Work out the finished part from the listing and answer in its coordinate system (mm). Face numbers are marked on the shaded views. A direction names the side the tool comes from. Coordinates: 2 decimals unless noted, no trailing zeros. Write each loop counter-clockwise with the first axis right and the second up, starting at its lowest first coordinate (ties: lowest second). Pieces come first, ordered by that corner, then holes. Notation, with made-up numbers: (40.25, 12) - (89.25, 12) arc R8 ccw to (89.25, 19) - close; hole circle Ø8 at (-34.5, -35). An arc over 180 degrees is marked (long way). One line per item, written item: value.
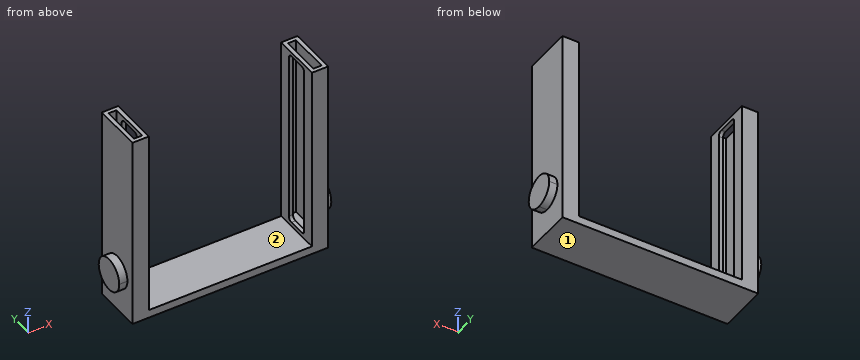
```python
from build123d import *

# Parameters (mm, degrees)
F0_W          = 25.4
F0_H          = 127
F1_DEPTH      = 31.75
F0_W_2        = 50.8
F0_H_2        = 152.4
F2_DEPTH      = 609.6
F0_W_3        = 508
F3_DEPTH      = 25.4
F4_DEPTH      = 609.6
F5_DEPTH      = 31.75
F6_W          = 76.2
F6_H          = 558.8
F7_DEPTH      = 25.4
F7_DEPTH_BACK = 533.4
F8_R          = 12.7
F10_DEPTH     = 25.4
F12_DEPTH     = 25.4


with BuildPart() as f1:
    # F0 (on Top) → F1 (new body)
    with BuildSketch(Plane.XY):
        with Locations((-80.5362447441, -59.7925535809)):
            Rectangle(F0_W, F0_H)
    extrude(amount=F1_DEPTH)

    # F0 (on Top) → F2 (join)
    with BuildSketch(Plane.XY):
        with Locations((-80.5362447441, -59.7925535809)):
            Rectangle(F0_W_2, F0_H_2)
        with Locations((-80.5362447441, -59.7925535809)):
            Rectangle(F0_W, F0_H, mode=Mode.SUBTRACT)
    extrude(amount=F2_DEPTH)

    # F0 (on Top) → F3 (join)
    with BuildSketch(Plane.XY):
        with Locations((198.8637552559, -59.7925535809)):
            Rectangle(F0_W_3, F0_H_2)
    extrude(amount=F3_DEPTH)

    # F0 (on Top) → F4 (join)
    with BuildSketch(Plane.XY):
        with Locations((478.2637552559, -59.7925535809)):
            Rectangle(F0_W_2, F0_H_2)
        with Locations((478.2637552559, -59.7925535809)):
            Rectangle(F0_W, F0_H, mode=Mode.SUBTRACT)
    extrude(amount=F4_DEPTH)

    # F0 (on Top) → F5 (join)
    with BuildSketch(Plane.XY):
        with Locations((478.2637552559, -59.7925535809)):
            Rectangle(F0_W, F0_H)
    extrude(amount=F5_DEPTH)

    # F6 (on face) → F7 (cut, two sides)
    with BuildSketch(Plane(origin=(452.8637552559, 0, 0), x_dir=(0, -1, 0), z_dir=(-1, 0, 0))) as f7_sk:
        with Locations((59.7925535809, 317.5)):
            Rectangle(F6_W, F6_H)
    extrude(amount=-F7_DEPTH, mode=Mode.SUBTRACT)
    extrude(f7_sk.sketch, amount=F7_DEPTH_BACK, mode=Mode.SUBTRACT)

    # F8
    f8_edges = [f1.edges().sort_by_distance(p)[0] for p in [
        (459.213755, -97.892554, 38.1),
        (459.213755, -21.692554, 38.1),
        (459.213755, -97.892554, 596.9),
        (459.213755, -21.692554, 596.9),
        (-61.486245, -21.692554, 38.1),
        (-61.486245, -21.692554, 596.9),
        (-61.486245, -97.892554, 596.9),
        (-61.486245, -97.892554, 38.1),
    ]]
    fillet(f8_edges, radius=F8_R)

    # F9 (on face) → F10 (join)
    with BuildSketch(Plane(origin=(-105.9362447441, 0, 0), x_dir=(0, -1, 0), z_dir=(-1, 0, 0))):
        with BuildLine():
            ThreePointArc((59.7925535809, 76.2), (95.7135780651, 91.0789755157), (110.5925535809, 127))
            ThreePointArc((110.5925535809, 127), (23.8715290966, 162.9210244843), (59.7925535809, 76.2))
        make_face()
    extrude(amount=F10_DEPTH)

    # F11 (on face) → F12 (join)
    with BuildSketch(Plane.YZ.offset(503.6637552559)):
        with BuildLine():
            ThreePointArc((-8.9925535809, 127), (-95.7135780651, 162.9210244843), (-59.7925535809, 76.2))
            ThreePointArc((-59.7925535809, 76.2), (-23.8715290966, 91.0789755157), (-8.9925535809, 127))
        make_face()
    extrude(amount=F12_DEPTH)


solid = f1.part
```
Item 1: Which of the six approach directions +Z, -Z, +X, -X, +Y, -Y give full straight-line access (tool end or side, diameter ignored) to the marked faces 1 and 2?
Evaluation:
face 1: -Z, +X, -X, +Y, -Y
face 2: +Z, +Y, -Y
Item 2: Section B-B, the plane x = 477.5 is taken. Determine the outline of the cut face in (y, z), then the cut area to 3 significant figures.
Evaluation:
outline: (-135.99, 0) - (16.41, 0) - (16.41, 609.6) - (3.71, 609.6) - (3.71, 31.75) - (-123.29, 31.75) - (-123.29, 609.6) - (-135.99, 609.6) - close
area: 19,500 mm2
Item 3: Given pin 1 (1 mm diameter, centred on y = -118, z = 431.5, fed in from -X); pin 2 (7.5 mm diameter, centred on x = 481, y = -49, fed in from +Z); pin 3 (1 mm diameter, centred on x = 421.5, y = -73.5, fed in from +Z), each flat-ended and moving along its own axis, determine where each tip first touches the part or whether it passes through.
Evaluation:
pin 1: stops at x = -105.94
pin 2: stops at z = 31.75
pin 3: stops at z = 25.4
Item 4: Section C-C, the plane y = -51.5 is taken. Give the number of separate pieces and of enclosed holes in the cut face, then the cut area to 3 significant figures.
Evaluation:
separate pieces: 3
enclosed holes: 0
area: 36,400 mm2
Item 5: Section D-D, the plane x = -22 is taken. Determine the outline of the cut face in (y, z), then the cut area to 3 significant figures.
Evaluation:
outline: (-135.99, 0) - (16.41, 0) - (16.41, 25.4) - (-135.99, 25.4) - close
area: 3,870 mm2
Item 6: Section A-A, the plane z = 403 is taken. Determine the outline of the cut face in (x, y), then the cut area to 3 significant figures.
Evaluation:
outline: (-105.94, -135.99) - (-55.14, -135.99) - (-55.14, -97.89) - (-67.84, -97.89) - (-67.84, -123.29) - (-93.24, -123.29) - (-93.24, 3.71) - (-67.84, 3.71) - (-67.84, -21.69) - (-55.14, -21.69) - (-55.14, 16.41) - (-105.94, 16.41) - close; (452.86, -135.99) - (503.66, -135.99) - (503.66, 16.41) - (452.86, 16.41) - (452.86, -21.69) - (465.56, -21.69) - (465.56, 3.71) - (490.96, 3.71) - (490.96, -123.29) - (465.56, -123.29) - (465.56, -97.89) - (452.86, -97.89) - close
area: 7,100 mm2
Item 7: Consider probe 1 along X at (y, z) = (-112, 335); probe 2 along X at (y, z) = (7, 429.5); probe 3 along X at (y, z) = (-89.5, 373). Determine where each line is inside the solid, lowest interval first.
Evaluation:
probe 1: x = -105.94 to -93.24, -67.84 to -55.14, 452.86 to 465.56, 490.96 to 503.66
probe 2: x = -105.94 to -55.14, 452.86 to 503.66
probe 3: x = -105.94 to -93.24, 490.96 to 503.66
